from build123d import *

# Parameters (mm, degrees)
BOSS_EXTRUDE2_DEPTH     = 26
CUT_EXTRUDE2_DEPTH      = 30.853140538
CUT_EXTRUDE2_DEPTH_BACK = 30.853140538
SKETCH2_R               = 1.2
SKETCH3_W               = 52
SKETCH3_H               = 13.4
BOSS_EXTRUDE3_DEPTH     = 1.5


with BuildPart() as part:
    # Sketch1 → Boss-Extrude2 (new, symmetric)
    with BuildSketch(Plane.XY):
        Polygon((0, 0), (6.1, 0), (6.1, 2.6), (13.6, 2.6), (13.6, 5.5), (0, 5.5), align=None)
    extrude(amount=BOSS_EXTRUDE2_DEPTH, both=True)

    # Sketch2 → Cut-Extrude2 (cut, two sides: drawn at the far end of the back side and taken through both)
    with BuildSketch(Plane(origin=(0, 0, 0), x_dir=(1, 0, 0), z_dir=(0, 1, 0)).offset(-CUT_EXTRUDE2_DEPTH_BACK)):
        with Locations(Location((2.7, 22, 0), (0, 0, 270))):
            Circle(SKETCH2_R)
        with Locations(Location((2.7, 0, 0), (0, 0, 270))):
            Circle(SKETCH2_R)
        with Locations(Location((2.7, -22, 0), (0, 0, 270))):
            Circle(SKETCH2_R)
    extrude(amount=CUT_EXTRUDE2_DEPTH + CUT_EXTRUDE2_DEPTH_BACK, mode=Mode.SUBTRACT)

    # Sketch3 → Boss-Extrude3 (add)
    with BuildSketch(Plane(origin=(13.6, 0, 0), x_dir=(0, 0, -1), z_dir=(1, 0, 0))):
        with Locations((0, 9.3)):
            Rectangle(SKETCH3_W, SKETCH3_H)
    extrude(amount=BOSS_EXTRUDE3_DEPTH)


solid = part.part
Input: part model. Units: mm. Frame: model coordinates. A direction names the side the tool comes from. Round coordinates to 2 decimals unless told otherwise and drop trailing zeros. Loops run counter-clockwise (first coordinate to the right, second up) from the corner with the lowest first, then second, coordinate; pieces in that order, holes last. Notation, with made-up numbers: M 55.5,-38.75 L 111.5,-38.75 A30 ccw 111.5,-1.75 Z; hole C 88.25,-8 d5. An arc over 180 degrees is marked long. Answer as CSV lines item,"result". Start each with the question number.
(1) Section A-A, the plane z = 0. Output: boundary loops of the cut face in (x, y).
(2) Draft query along Z for faces 4 (the flat face through (11, 2.6, 0)), 5 (the flat face through (8, 5, -26)), 6 (the cylindrical face through (1.97, 2.71, -22.95)), 7 (the cylindrical face through (1.97, 2.71, 21.05)). Return one class per face: released by +Z, released by -Z, zero draft, split by the parting line, or undercut.
(3) First-contact query: pin 1 (1.3 mm diameter, centred on y = 2, z = -7, fed in from +X); pin 2 (4.5 mm diameter, centred on x = 13, z = -5, fed in from -Y); pin 3 (5 mm diameter, centred on y = 10, z = 18.5, fed in from -X); pin 4 (2 mm diameter, centred on x = 10, z = -2, fed in from +Y). Flat tips, straight axial feed; report the tip coordinate or a pass-through.
(4) Section C-C, the plane y = 4.75. Output: boundary loops of the cut face in (x, z), plus the area to 3 significant figures.
(5) Reachability of faces 1 (the flat face through (8, 5, 26)), 2 (the flat face through (7, 5.5, 0)), 3 (the flat face through (6.1, 1, 0)) from +Z, -Z, +X, -X, +Y, -Y: full face, straight path, thin tool, end or side. Return the list, or none.
(6) Section D-D, the plane z = 7. Output: boundary loops of the cut face in (x, y), plus the area to 3 significant figures.
(7) Line query: line 1 (Z direction, x = 2.7, y = 1.55); line 2 (X direction, y = 3.35, z = -22); line 3 (X direction, y = 2.05, z = 22). Output: solid intervals per line, ascending. Write a range as [from, to].
(8) Section B-B, the plane x = 2.7. Output: boundary loops of the cut face in (y, z), plus the area to 3 significant figures.
Values found:
1,outline,"M 0,0 L 1.5,0 L 1.5,5.5 L 0,5.5 Z; M 3.9,0 L 6.1,0 L 6.1,2.6 L 15.1,2.6 L 15.1,16 L 13.6,16 L 13.6,5.5 L 3.9,5.5 Z"
2,face 4,"zero draft"
2,face 5,"released by -Z"
2,face 6,"undercut"
2,face 7,"undercut"
3,pin 1,"stops at x = 15.1"
3,pin 2,"stops at y = 2.6"
3,pin 3,"stops at x = 13.6"
3,pin 4,"stops at y = 5.5"
4,outline,"M 0,-26 L 15.1,-26 L 15.1,26 L 0,26 Z; hole C 2.7,-22 d2.4; hole C 2.7,0 d2.4; hole C 2.7,22 d2.4"
4,area,"772 mm²"
5,face 1,"+Z, +X, -X, +Y, -Y"
5,face 2,"+Z, -Z, -X, +Y"
5,face 3,"+Z, -Z, +X, -Y"
6,outline,"M 0,0 L 6.1,0 L 6.1,2.6 L 15.1,2.6 L 15.1,16 L 13.6,16 L 13.6,5.5 L 0,5.5 Z"
6,area,"75.4 mm²"
7,line 1,"z = [-26, -23.2], [-20.8, -1.2], [1.2, 20.8], [23.2, 26]"
7,line 2,"x = [0, 1.5], [3.9, 15.1]"
7,line 3,"x = [0, 1.5], [3.9, 6.1]"
8,outline,"M 0,-26 L 5.5,-26 L 5.5,-23.2 L 0,-23.2 Z; M 0,-20.8 L 5.5,-20.8 L 5.5,-1.2 L 0,-1.2 Z; M 0,1.2 L 5.5,1.2 L 5.5,20.8 L 0,20.8 Z; M 0,23.2 L 5.5,23.2 L 5.5,26 L 0,26 Z"
8,area,"246 mm²"
